from build123d import *

# Parameters (mm, degrees)
F0_R     = 10
F1_DEPTH = 5
F2_R     = 5.25
F3_DEPTH = 5.001
F6_DEPTH = 50


with BuildPart() as f1:
    # F0 (on Top) → F1 (new body)
    with BuildSketch(Plane.XY):
        Circle(F0_R)
    extrude(amount=F1_DEPTH)

    # F2 (on face) → F3 (cut, through all)
    with BuildSketch(Plane.XY.offset(5)):
        Circle(F2_R)
    extrude(amount=-F3_DEPTH, mode=Mode.SUBTRACT)

    # F5 (on offset) → F6 (cut)
    with BuildSketch(Plane.XZ.offset(25)):
        Polygon((-11.632799, 5.720356), (-23.740912, 0), (45.850801, 5.720356), align=None)
    extrude(amount=-F6_DEPTH, mode=Mode.SUBTRACT)


solid = f1.part
Source: CAD feature listing. Evaluate the final solid. Frame: model axes, mm. Coordinates: 2 decimals unless noted, no trailing zeros. Loops run counter-clockwise (first coordinate to the right, second up) from the corner with the lowest first, then second, coordinate; pieces in that order, holes last. Notation, with made-up numbers: M 33.25,3.25 L 83.25,3.25 A15 cw 83.25,8.25 Z; hole C 24.5,-9.75 d9. An arc over 180 degrees is marked long. Answer in a Markdown table with one row per item.
Q1. Section D-D on y = -6.5. Return the cut outline in (x, z).
Answers below:
| item | result |
|---|---|
| outline | M -7.6,0 L 7.6,0 L 7.6,2.58 L -7.6,1.33 Z |
Q2. First-contact query: pin 1 (1.5 mm diameter, centred on y = -7, z = 0.5, fed in from -X); pin 2 (10 mm diameter, centred on x = 0.5, y = -3, fed in from +Z). Flat tips, straight axial feed; report the tip coordinate or a pass-through.
Answers below:
| item | result |
|---|---|
| pin 1 | stops at x = -7.81 |
| pin 2 | stops at z = 2.4 |
Q3. Section C-C on z = 0.4. Return the cut outline in (x, y).
Answers below:
| item | result |
|---|---|
| outline | C 0,0 d20; hole C 0,0 d10.5 |
Q4. Section A-A on y = 0. Return the cut outline in (x, z), plus the area to 3 significant figures.
Answers below:
| item | result |
|---|---|
| outline | M -10,0 L -5.25,0 L -5.25,1.52 L -10,1.13 Z; M 5.25,0 L 10,0 L 10,2.77 L 5.25,2.38 Z |
| area | 18.5 mm^2 |
Q5. Ray query, probe 1 along Y at (x, z) = (0, 0.9); probe 2 along X at (y, z) = (3, 0.75). Return the intervals inside material, ascending. Write a range as from..to.
Answers below:
| item | result |
|---|---|
| probe 1 | y = -10..-5.25, 5.25..10 |
| probe 2 | x = -9.54..-4.31, 4.31..9.54 |
Q6. Section B-B on x = 0. Return the cut outline in (y, z), plus the area to 3 significant figures.
Answers below:
| item | result |
|---|---|
| outline | M -10,0 L -5.25,0 L -5.25,1.95 L -10,1.95 Z; M 5.25,0 L 10,0 L 10,1.95 L 5.25,1.95 Z |
| area | 18.5 mm^2 |
Q7. Draft query along X for faces 1 (the cylindrical face through (5, 1.6, 0.9)), 2 (the flat face through (4.304, 4.304, 2.305)), 3 (the flat face through (4, -4, 0)). Return one class per face: pulls with the +X half, pulls with the -X half, needs draft (parallel to the pull), parting line crosses it, or undercut.
Answers below:
| item | result |
|---|---|
| face 1 | undercut |
| face 2 | pulls with the -X half |
| face 3 | needs draft |
